Autodesk Inventor part; units mm, degrees
ref_plane "YZ Plane" through (0, 0, 0) normal (1, 0, 0) x (0, 1, 0)
ref_plane "XZ Plane" through (0, 0, 0) normal (0, 1, 0) x (-1, 0, 0)
ref_plane "XY Plane" through (0, 0, 0) normal (0, 0, 1) x (1, 0, 0)
sketch "Sketch2" plane through (0, 0, 0) normal (0, 1, 0) x (-1, 0, 0)
  line L0 (0, 0) -> (-60, 0)
  line L1 (-60, 0) -> (-60, -20)
  line L2 (-60, -20) -> (0, -20)
  line L3 (0, -20) -> (0, 0)
  line L4 (0, -20) -> (-20, -20)
  line L5 (-20, -20) -> (-20, -60)
  line L6 (-20, -60) -> (0, -60)
  line L7 (0, -60) -> (0, -20)
  line L8 (-20, -20) -> (-35, -20)
  line L9 (-20, -20) -> (-20, -35)
  line L10 (-60, -20) -> (-20, -60)
  line L11 (-60, 0) -> (-60, -10)
  line L12 (-60, -10) -> (-50, -10)
  circle A0 centre (-50, -10) radius 2.5
  circle A1 centre (-30, -10) radius 2.5
  circle A2 centre (-10, -10) radius 2.5
  circle A3 centre (-10, -30) radius 2.5
  line L13 (0, -80) -> (0, -40)
  circle A4 centre (-10, -50) radius 2.5
  line L14 (0, -100) -> (0, -60)
  dimension "d4" = 60
  dimension "d5" = 20
  dimension "d6" = 20
  dimension "d7" = 40
  dimension "d10" = 10
  dimension "d11" = 10
  dimension "d12" = 5
  dimension "d15" = 20
  dimension "d22" = 20
extrude "Extrusion1" add sketch "Sketch2" against normal blind 2
properties part number "Connect2x2020_m5" material "Aluminum 6061"
The listing builds one solid part. Answer for the finished solid, in the listing's coordinates (mm). Give positions to 0.01 mm unless a question says otherwise; leave off trailing zeros. Order: outer loops, then holes, each group sorted by start corner. A loop starts at its lowest first (then second) coordinate and runs counter-clockwise, first axis right, second up. Notation, with made-up numbers: (33, 49) - (65, 49) arc R28 ccw to (65, 81) - close; hole circle Ø8 at (-4, 35). An arc over 180 degrees is marked (long way). Use one line per item in the form item = value. Start each with the question number.
(1) The mould has two halves that part along Z. Classify faces 1 (the flat face through (0, -1, -30)), 2 (the cylindrical face through (47.69, -0.99, -10.96)), 3 (the flat face through (10, -1, -60)): released by +Z, released by -Z, zero draft, split by the parting line, or undercut.
(2) A cutting plane is placed at B-B, the plane z = -50. Write down the section's boundary in (x, y), then the cut area to 3 significant figures.
(3) A cutting plane is placed at C-C, the plane y = -1.05. Write down the section's boundary in (x, z).
(4) A cutting plane is placed at A-A, the plane x = 30. Write down the section's boundary in (y, z).
(5) A cutting plane is placed at D-D, the plane z = -10. Write down the section's boundary in (x, y).
(6) Consider line 1 (Z direction, x = 10, y = -1.3); line 2 (X direction, y = -1, z = -11); line 3 (Z direction, x = 11.5, y = -1.7). Determine where each line is inside the solid, lowest interval first. Write a range as from..to.
Ans:
q1.face_1 = zero draft
q1.face_2 = undercut
q1.face_3 = released by -Z
q2.outline = (0, -2) - (7.5, -2) - (7.5, 0) - (0, 0) - close; (12.5, -2) - (30, -2) - (30, 0) - (12.5, 0) - close
q2.area = 50.0 mm^2
q3.outline = (0, -60) - (20, -60) - (60, -20) - (60, 0) - (0, 0) - close; hole circle Ø5 at (10, -50); hole circle Ø5 at (10, -30); hole circle Ø5 at (10, -10); hole circle Ø5 at (30, -10); hole circle Ø5 at (50, -10)
q4.outline = (-2, -50) - (0, -50) - (0, -12.5) - (-2, -12.5) - close; (-2, -7.5) - (0, -7.5) - (0, 0) - (-2, 0) - close
q5.outline = (0, -2) - (7.5, -2) - (7.5, 0) - (0, 0) - close; (12.5, -2) - (27.5, -2) - (27.5, 0) - (12.5, 0) - close; (32.5, -2) - (47.5, -2) - (47.5, 0) - (32.5, 0) - close; (52.5, -2) - (60, -2) - (60, 0) - (52.5, 0) - close
q6.line_1 = -60..-52.5, -47.5..-32.5, -27.5..-12.5, -7.5..0
q6.line_2 = 0..7.71, 12.29..27.71, 32.29..47.71, 52.29..60
q6.line_3 = -60..-52, -48..-32, -28..-12, -8..0
